Here's how the part is built. I have some questions about the finished solid (model axes, mm). Face numbers are marked on the shaded views. A direction names the side the tool comes from. Give positions to 0.01 mm unless a question says otherwise; leave off trailing zeros. Loops run counter-clockwise (first coordinate to the right, second up) from the corner with the lowest first, then second, coordinate; pieces in that order, holes last. Notation, with made-up numbers: M 13.25,76.25 L 64.25,76.25 A28 cw 64.25,100.25 Z; hole C 27.25,-1.75 d2. An arc over 180 degrees is marked long. Answer as CSV lines item,"result". Start each with the question number.
Item 1: I want a section at D-D on x = 33. List the corners of the cut face in (y, z) for me.
Item 2: I want a section at B-B on y = 0. List the corners of the cut face in (x, z) for me.
Item 3: Will these pins go through, and if not, where does the flat tip stop? P1, Ø1, axis at y = 5, z = -0.5, coming from the -X side; P2, Ø6, axis at x = 26.5, z = 2.5, coming from the +Y side; P3, Ø8, axis at x = 25.5, z = 0.5, coming from the -Y side.
Item 4: For the marked faces 1 and 2, which set-ups out of +Z, -Z, +X, -X, +Y, -Y let a thin tool reach every point of the face, with its end or its side?
Item 5: If I drill on line 1 along Y through (x, z) = (20.5, 0.25); line 2 along X through (y, z) = (-4.5, -3.75); line 3 along Z through (x, y) = (0.5, 3), over which ranges is the centre line in solid material (lowest first)? Write a range as from..to.
Item 6: I want a section at A-A on z = 0. List the corners of the cut face in (x, y) for me, plus the area to 3 significant figures.
Item 7: I want a section at C-C on x = -9. List the corners of the cut face in (y, z) for me.
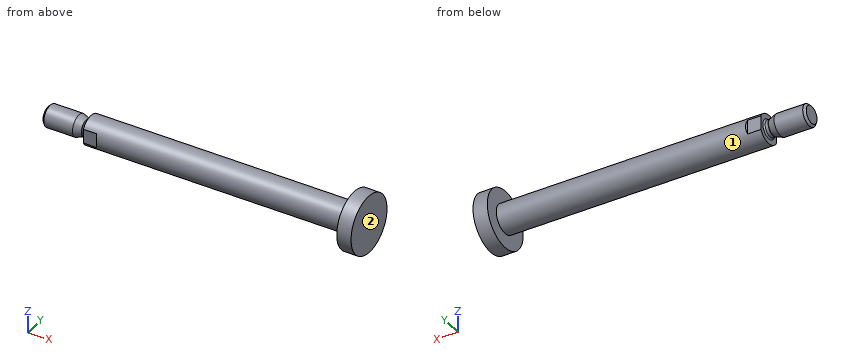
Autodesk Inventor part; units mm, degrees
ref_plane "FDT_PIRODACC_M1_XY" through (-10.9, 0, 0) normal (-1, 0, 0) x (0, 1, 0)
ref_plane "FDT_PIRODACC_M1_YZ" through (-10.9, 0, 0) normal (0, 1, 0) x (0, 0, -1)
ref_plane "FDT_PIRODACC_M1_ZX" through (-10.9, 0, 0) normal (0, 0, -1) x (-1, 0, 0)
sketch "Sketch_1" plane through (0, 0, 0) normal (0, 0, 1) x (1, 0, 0)
  line L0 (73, 0) -> (-4.7, 0)
  line L1 (-4.7, 0) -> (-4.7, 4)
  line L2 (-4.7, 4) -> (73, 4)
  line L3 (73, 4) -> (73, 0)
  line L4 (73, 0) -> (-4.7, 0)
revolve "Revolution1" add sketch "Sketch_1" angle 360 about axis through (73, 0, 0) along (1, 0, 0)
sketch "Sketch_11" plane through (0, 0, 0) normal (0, 0, 1) x (1, 0, 0)
  line L0 (73, 0) -> (69, 0)
  line L1 (69, 0) -> (69, 8)
  line L2 (69, 8) -> (73, 8)
  line L3 (73, 8) -> (73, 0)
  line L4 (73, 0) -> (69, 0)
revolve "Revolution2" add sketch "Sketch_11" angle 360 about axis through (73, 0, 0) along (1, 0, 0)
sketch "Sketch_19" plane through (0, 0, 0) normal (0, 0, 1) x (1, 0, 0)
  line L0 (-3.7, 0) -> (-16.7, 0)
  line L1 (-16.7, 0) -> (-16.7, 2.3865)
  line L2 (-16.7, 2.3865) -> (-16.0865, 3)
  line L3 (-16.0865, 3) -> (-8.0606, 3)
  line L4 (-8.0606, 3) -> (-6.0663, 2.2741)
  arc A0 (-6.0663, 2.2741) -> (-5.9295, 2.25) centre (-5.9295, 2.65) ccw
  line L5 (-5.9295, 2.25) -> (-5.1, 2.25)
  arc A1 (-5.1, 2.25) -> (-4.7, 2.65) centre (-5.1, 2.65) ccw
  line L6 (-4.7, 2.65) -> (-4.7, 3)
  line L7 (-4.7, 3) -> (-3.7, 3)
  line L8 (-3.7, 3) -> (-3.7, 0)
  line L9 (-3.7, 0) -> (-16.7, 0)
revolve "Revolution3" add sketch "Sketch_19" angle 360 about axis through (-3.7, 0, 0) along (1, 0, 0)
thread "Thread1"
sketch "Sketch_20" plane through (0, 0, 0) normal (0, 0, 1) x (1, 0, 0)
  line L0 (-26.4, -12.5) -> (4.1962, -12.5)
  line L1 (4.1962, -12.5) -> (-1, -3.5)
  line L2 (-1, -3.5) -> (-4.7, -3.5)
  line L3 (-4.7, -3.5) -> (-4.7, -8.5)
  line L4 (-4.7, -8.5) -> (-21.7, -8.5)
  line L5 (-21.7, -8.5) -> (-21.7, 8.5)
  line L6 (-21.7, 8.5) -> (-4.7, 8.5)
  line L7 (-4.7, 8.5) -> (-4.7, 3.5)
  line L8 (-4.7, 3.5) -> (-1, 3.5)
  line L9 (-1, 3.5) -> (4.1962, 12.5)
  line L10 (4.1962, 12.5) -> (-26.4, 12.5)
  line L11 (-26.4, 12.5) -> (-26.4, -12.5)
extrude "Extrusion1" cut sketch "Sketch_20" along normal mid plane 16
ref_plane "FDT_PIRODACC_M1_XY" through (-10.9, 0, 0) normal (-1, 0, 0) x (0, 1, 0)
ref_plane "FDT_PIRODACC_M1_YZ" through (-10.9, 0, 0) normal (0, 1, 0) x (0, 0, -1)
ref_plane "FDT_PIRODACC_M1_ZX" through (-10.9, 0, 0) normal (0, 0, -1) x (-1, 0, 0)
ref_plane "NUT1_XY" through (-9.3, 0, 0) normal (1, 0, 0) x (0, 0, -1)
ref_plane "NUT1_YZ" through (-9.3, 0, 0) normal (0, 0, -1) x (0, 1, 0)
ref_plane "NUT1_ZX" through (-9.3, 0, 0) normal (0, 1, 0) x (1, 0, 0)
ref_plane "PISTON_XY" through (73, 0, 0) normal (1, 0, 0) x (0, 0, -1)
ref_plane "PISTON_YZ" through (73, 0, 0) normal (0, 0, -1) x (0, 1, 0)
ref_plane "PISTON_ZX" through (73, 0, 0) normal (0, 1, 0) x (1, 0, 0)
properties part number "536218 ADN-50-P-A_(KS)"
Result:
1,outline,"C 0,0 d8"
2,outline,"M -16.7,-2.39 L -16.09,-3 L -8.06,-3 L -6.07,-2.27 A0.4 cw -5.93,-2.25 L -5.1,-2.25 A0.4 cw -4.7,-2.65 L -4.7,-4 L 69,-4 L 69,-8 L 73,-8 L 73,8 L 69,8 L 69,4 L -4.7,4 L -4.7,2.65 A0.4 cw -5.1,2.25 L -5.93,2.25 A0.4 cw -6.07,2.27 L -8.06,3 L -16.09,3 L -16.7,2.39 Z"
3,P1,"x = 69"
3,P2,"y = 4"
3,P3,"y = -4"
4,face 1,"-X"
4,face 2,"+Z, -Z, +X, +Y, -Y"
5,line 1,"-3.99..3.99"
5,line 2,"69..73"
5,line 3,"-2.65..2.65"
6,outline,"M -16.7,-2.39 L -16.09,-3 L -8.06,-3 L -6.07,-2.27 A0.4 cw -5.93,-2.25 L -5.1,-2.25 A0.4 cw -4.7,-2.65 L -4.7,-3.5 L -1,-3.5 L -0.71,-4 L 69,-4 L 69,-8 L 73,-8 L 73,8 L 69,8 L 69,4 L -0.71,4 L -1,3.5 L -4.7,3.5 L -4.7,2.65 A0.4 cw -5.1,2.25 L -5.93,2.25 A0.4 cw -6.07,2.27 L -8.06,3 L -16.09,3 L -16.7,2.39 Z"
6,area,"718 mm^2"
7,outline,"C 0,0 d6"
